```python
from build123d import *

# Parameters (mm, degrees)
SKETCH1_W                 = 6.7056
SKETCH1_H                 = 6.5278
SKETCH1_W_2               = 6.5278
BOSS_EXTRUDE1_DEPTH       = 3.175
F_6_CLEARANCE_HOLE1_D     = 3.7973
F_6_CLEARANCE_HOLE1_DEPTH = 6.35
F_6_CLEARANCE_HOLE1_TIP   = 1.140824014
FILLET1_R                 = 1.27


with BuildPart() as part:
    # Sketch1 → Boss-Extrude1 (new body)
    with BuildSketch(Plane(origin=(0, 0, 0), x_dir=(1, 0, 0), z_dir=(0, 1, 0))):
        Polygon((127.426380641, 27.563643867), (15.082180641, 27.563643867), (15.082180641, 22.623343867), (8.198780641, 22.623343867), (8.198780641, 27.208043867), (-9.225619359, 27.208043867), (-9.225619359, 23.575843867), (-15.575619359, 23.575843867), (-15.575619359, 15.993943867), (-9.225619359, 15.993943867), (-9.225619359, 9.110543867), (-15.575619359, 9.110543867), (-15.575619359, 1.706443867), (0.1397, 1.706443867), (0.1397, 0.118943867), (15.082180641, 0.118943867), (15.082180641, -0.058856133), (127.426380641, -0.058856133), (127.426380641, 0.118943867), (142.191061281, 0.118943867), (142.191061281, 1.528643867), (157.906380641, 1.528643867), (157.906380641, 9.110543867), (151.556380641, 9.110543867), (151.556380641, 15.993943867), (157.906380641, 15.993943867), (157.906380641, 23.575843867), (151.556380641, 23.575843867), (151.556380641, 27.208043867), (134.131980641, 27.208043867), (134.131980641, 22.623343867), (127.426380641, 22.623343867), align=None)
        with Locations((11.729380641, 6.075243867)):
            Rectangle(SKETCH1_W, SKETCH1_H, mode=Mode.SUBTRACT)
        Polygon((68.349676501, 2.303343867), (17.444380641, 2.303343867), (17.444380641, 25.023643867), (23.391676501, 25.023643867), align=None, mode=Mode.SUBTRACT)
        with Locations((130.690280641, 6.075243867)):
            Rectangle(SKETCH1_W_2, SKETCH1_H, mode=Mode.SUBTRACT)
        Polygon((73.981084781, 2.303343867), (118.939084781, 25.023643867), (124.886380641, 25.023643867), (124.886380641, 2.303343867), align=None, mode=Mode.SUBTRACT)
        Polygon((-6.228419359, 8.001876918), (-6.228419359, 22.168725531), (3.653156436, 8.001876918), align=None, mode=Mode.SUBTRACT)
        Polygon((-4.679995154, 24.388643867), (5.201580641, 24.388643867), (5.201580641, 10.221795255), align=None, mode=Mode.SUBTRACT)
        Polygon((113.307676501, 25.023643867), (71.165380641, 3.726308474), (29.023084781, 25.023643867), align=None, mode=Mode.SUBTRACT)
        Polygon((148.559180641, 22.168725531), (148.559180641, 8.001876918), (138.677604846, 8.001876918), align=None, mode=Mode.SUBTRACT)
        Polygon((137.129180641, 24.388643867), (147.010756436, 24.388643867), (137.129180641, 10.221795255), align=None, mode=Mode.SUBTRACT)
    extrude(amount=BOSS_EXTRUDE1_DEPTH)

    # #6 Clearance Hole1
    with Locations(Plane(origin=(0.024087856, 3.175, -12.509508824), x_dir=(-1, 0, 0), z_dir=(0, 1, 0))):
        with Locations((-130.577292784, -6.164135043), (-154.707292784, -7.499674703), (-154.707292784, 6.787825297), (-11.737042784, -6.164130843), (12.392957216, 6.787829497), (12.462807216, -7.499674703)):
            Hole(F_6_CLEARANCE_HOLE1_D / 2, depth=F_6_CLEARANCE_HOLE1_DEPTH)
            with Locations((0, 0, -(F_6_CLEARANCE_HOLE1_DEPTH + F_6_CLEARANCE_HOLE1_TIP / 2))):  # 118° drill point
                Cone(0, F_6_CLEARANCE_HOLE1_D / 2, F_6_CLEARANCE_HOLE1_TIP, mode=Mode.SUBTRACT)

    # Fillet1
    fillet1_edges = [part.edges().sort_by_distance(p)[0] for p in [
        (-6.228419359, 1.5875, -22.168725531),
        (-6.228419359, 1.5875, -8.001876918),
        (3.653156436, 1.5875, -8.001876918),
        (124.886380641, 1.5875, -2.303343867),
        (73.981084781, 1.5875, -2.303343867),
        (17.444380641, 1.5875, -2.303343867),
        (138.677604846, 1.5875, -8.001876918),
        (148.559180641, 1.5875, -8.001876918),
        (148.559180641, 1.5875, -22.168725531),
        (137.129180641, 1.5875, -24.388643867),
        (137.129180641, 1.5875, -10.221795255),
        (147.010756436, 1.5875, -24.388643867),
        (5.201580641, 1.5875, -10.221795255),
        (5.201580641, 1.5875, -24.388643867),
        (-4.679995154, 1.5875, -24.388643867),
    ]]
    fillet(fillet1_edges, radius=FILLET1_R)


solid = part.part
```
For this review, take the finished solid that the model builds, in its own axes (mm). A direction names the side the tool comes from. Round coordinates to 2 decimals unless told otherwise and drop trailing zeros. Write each loop counter-clockwise with the first axis right and the second up, starting at its lowest first coordinate (ties: lowest second). Pieces come first, ordered by that corner, then holes. Notation, with made-up numbers: M 78,54.5 L 105,54.5 A14 ccw 105,63.5 Z; hole C 49.5,22.25 d4. An arc over 180 degrees is marked long. One line per item, written item: value. Start each with the question number.
(1) Wall thickness on line 1 (Z direction, x = 2, y = 2.8); line 2 (X direction, y = 2.65, z = -10); line 3 (Z direction, x = 82, y = 1.85): over which ranges is each line inside the solid? List them lowest first.
(2) The part is to be moulded in two halves that separate along X. For faces 4 (the flat face through (157.906, 2, -20)), 5 (the flat face through (-12, 2, -9.111)), 6 (the flat face through (44, 2, -2.303)), say which applies: released by +X, released by -X, zero draft, split by the parting line, or undercut.
(3) Insertion check: pin 1 (5 mm diameter, centred on x = 49.5, z = -18, fed in from +Y); pin 2 (1 mm diameter, centred on x = 6.5, y = 1, fed in from +Z); pin 3 (1.6 mm diameter, centred on y = 1.5, z = -13, fed in from +X); pin 4 (1.5 mm diameter, centred on x = 109, z = -20, fed in from -Y). Each pin has a flat end and moves straight along its axis. Give the tip position at first contact, or say it passes through.
(4) Machinability: for faces 1 (the flat face through (12, 2, -22.623)), 2 (the flat face through (-9.226, 2, -25)), 3 (the flat face through (-0.155, 1.565, -17.902)), which of the approach directions +Z, -Z, +X, -X, +Y, -Y give a long, thin tool a straight path to every point of the face, cutting with its end or side? Answer none if there is none.
(5) We need section B-B (y = 1.7). Count the separate pieces of the cut face and the enclosed holes in it, and give its area (3 significant figures).
(6) We need section A-A (x = 44.5). Give the boundary of the cut face in (y, z) (3 decimals), and give its area (3 significant figures).
Result:
1. line 1: -27.21 to -24.39, -14.81 to -10.37, -8.27 to -0.12
1. line 2: -9.23 to -6.23, 2.26 to 17.44, 53.12 to 58.75, 83.58 to 89.21, 124.89 to 140.07, 148.56 to 151.56
1. line 3: -27.56 to -25.02, -9.2 to -6.36, -2.3 to 0.06
2. face 4: released by +X
2. face 5: zero draft
2. face 6: undercut
3. pin 1: through
3. pin 2: z = -0.12
3. pin 3: x = 151.56
3. pin 4: y = 0
4. face 1: -Z, +Y, -Y
4. face 2: -Z, -X, +Y, -Y
4. face 3: +Y, -Y
5. separate pieces: 1
5. enclosed holes: 15
5. area: 1,920 mm²
6. outline: M 0,-27.564 L 3.175,-27.564 L 3.175,-25.024 L 0,-25.024 Z; M 0,-17.202 L 3.175,-17.202 L 3.175,-14.356 L 0,-14.356 Z; M 0,-2.303 L 3.175,-2.303 L 3.175,0.059 L 0,0.059 Z
6. area: 24.6 mm²
